Build history of the part. All positions in model axes, mm. A direction names the side the tool comes from. Round coordinates to 2 decimals unless told otherwise and drop trailing zeros. Write each loop counter-clockwise with the first axis right and the second up, starting at its lowest first coordinate (ties: lowest second). Pieces come first, ordered by that corner, then holes. Notation, with made-up numbers: (-35.5, -20.5) - (2.5, -20.5) arc R23 ccw to (2.5, 9.5) - close; hole circle Ø1 at (33, 21.5). An arc over 180 degrees is marked (long way). Write each question's results on one line, items separated by ' | '.
from build123d import *

# Parameters (mm, degrees)
F0_W     = 62
F0_H     = 62
F1_DEPTH = 2
F0_W_2   = 65
F0_H_2   = 65
F2_DEPTH = 50
F3_R     = 2
F4_R     = 1.8
F5_DEPTH = 25
F6_DEPTH = 25
F4_R_2   = 2.55
F7_DEPTH = 5


# Not quite as in the source:
# - a fillet or chamfer that OpenCascade refuses, or shapes differently, is made with other operations: its cross-section is extruded or revolved along the edge and cut away or added


with BuildPart() as f1:
    # F0 (on Front) → F1 (new body)
    with BuildSketch(Plane.XZ):
        with Locations((-0.6578962505, -3.6181825721)):
            Rectangle(F0_W, F0_H)
    extrude(amount=F1_DEPTH)

    # F0 (on Front) → F2 (join)
    with BuildSketch(Plane.XZ):
        with Locations((-0.6578962505, -3.6181825721)):
            Rectangle(F0_W_2, F0_H_2)
        with Locations((-0.6578962505, -3.6181825721)):
            Rectangle(F0_W, F0_H, mode=Mode.SUBTRACT)
    extrude(amount=F2_DEPTH)

    # F3
    f3_edges = [f1.edges().sort_by_distance(p)[0] for p in [
        (31.842104, 0, -3.618183),
        (-0.657896, 0, 28.881817),
        (-33.157896, 0, -3.618183),
        (-0.657896, 0, -36.118183),
        (31.842104, -25, 28.881817),
        (31.842104, -25, -36.118183),
        (-33.157896, -25, -36.118183),
        (-33.157896, -25, 28.881817),
    ]]
    fillet(f3_edges, radius=F3_R)

    # F4 (on face) → F5 (cut)
    with BuildSketch(Plane.YZ.offset(31.8421037495)):
        with Locations((-26, 21.3318174279)):
            Circle(F4_R)
    extrude(amount=-F5_DEPTH, mode=Mode.SUBTRACT)

    # F4 (on face) → F6 (cut)
    with BuildSketch(Plane.YZ.offset(31.8421037495)):
        with Locations((-26, 13.2318174279)):
            Circle(F4_R)
        with Locations((-26, 5.1318174279)):
            Circle(F4_R)
    extrude(amount=-F6_DEPTH, mode=Mode.SUBTRACT)

    # F4 (on face) → F7 (join)
    with BuildSketch(Plane.YZ.offset(31.8421037495)):
        with Locations((-26, 21.3318174279)):
            Circle(F4_R_2)
        with Locations((-26, 21.3318174279)):
            Circle(F4_R, mode=Mode.SUBTRACT)
        with Locations((-26, 13.2318174279)):
            Circle(F4_R_2)
        with Locations((-26, 13.2318174279)):
            Circle(F4_R, mode=Mode.SUBTRACT)
        with Locations((-26, 5.1318174279)):
            Circle(F4_R_2)
        with Locations((-26, 5.1318174279)):
            Circle(F4_R, mode=Mode.SUBTRACT)
    extrude(amount=F7_DEPTH)

    # F8: fillet of radius 1 on 3 edges, made by hand

    # F8_s1 → F8_t2 (revolve, cut)
    with BuildSketch(Plane.XY.offset(21.3318174279)):
        with BuildLine():
            ThreePointArc((35.873857913, -23.45), (36.4862303487, -23.659430585), (36.8421037495, -24.2))
            Line((36.8421037495, -24.2), (36.8421037495, -23.45))
            Line((36.8421037495, -23.45), (35.873857913, -23.45))
        make_face()
    revolve(axis=Axis((36.8421037495, -26, 21.3318174279), (1, 0, 0)), mode=Mode.SUBTRACT)

    # F8_s3 → F8_t4 (revolve, cut)
    with BuildSketch(Plane.XY.offset(13.2318174279)):
        with BuildLine():
            ThreePointArc((35.873857913, -23.45), (36.4862303487, -23.659430585), (36.8421037495, -24.2))
            Line((36.8421037495, -24.2), (36.8421037495, -23.45))
            Line((36.8421037495, -23.45), (35.873857913, -23.45))
        make_face()
    revolve(axis=Axis((36.8421037495, -26, 13.2318174279), (1, 0, 0)), mode=Mode.SUBTRACT)

    # F8_s5 → F8_t6 (revolve, cut)
    with BuildSketch(Plane.XY.offset(5.1318174279)):
        with BuildLine():
            ThreePointArc((35.873857913, -23.45), (36.4862303487, -23.659430585), (36.8421037495, -24.2))
            Line((36.8421037495, -24.2), (36.8421037495, -23.45))
            Line((36.8421037495, -23.45), (35.873857913, -23.45))
        make_face()
    revolve(axis=Axis((36.8421037495, -26, 5.1318174279), (1, 0, 0)), mode=Mode.SUBTRACT)


solid = f1.part
(1) Two-plate mould, pull along X, no slides. Class faces 1 (the flat face through (31.842, -26, -4)), 2 (the flat face through (-31.658, -26, -4)), 3 (the cylindrical face through (-0.231, -0.601, -35.548)): released by +X, released by -X, zero draft, split by the parting line, or undercut.
Worked answers:
face 1: released by +X | face 2: undercut | face 3: zero draft
(2) Slice it at B-B, the plane x = -27. Write the cut outline in (y, z), and give its area (3 significant figures).
Worked answers:
outline: (-50, -36.12) - (-2, -36.12) arc R2 ccw to (0, -34.12) - (0, 26.88) arc R2 ccw to (-2, 28.88) - (-50, 28.88) - (-50, 27.38) - (-2, 27.38) - (-2, -34.62) - (-50, -34.62) - close | area: 272 mm2
(3) Tool access for faces 4 (the cylindrical face through (33.83, -28.548, 21.444)), 5 (the cylindrical face through (31.24, -0.57, -3.19)), 6 (the flat face through (-1, -2, -3)): list every direction of +Z, -Z, +X, -X, +Y, -Y with a clear straight run to the whole face (end or side of a thin tool).
Worked answers:
face 4: +X | face 5: +Z, -Z, +X, +Y | face 6: -Y
(4) Slice it at D-D, the plane y = -26. State how many separate pieces and enclosed holes the cut face has, and give its area (3 significant figures).
Worked answers:
separate pieces: 3 | enclosed holes: 0 | area: 383 mm2
(5) Slice it at C-C, the plane z = 1. Write the cut outline in (x, y).
Worked answers:
outline: (-33.16, -50) - (-31.66, -50) - (-31.66, -2) - (30.34, -2) - (30.34, -50) - (31.84, -50) - (31.84, -2) arc R2 ccw to (29.84, 0) - (-31.16, 0) arc R2 ccw to (-33.16, -2) - close
(6) Slice it at A-A, the plane y = -16. Write the cut outline in (x, z), and give its area (3 significant figures).
Worked answers:
outline: (-33.16, -34.12) arc R2 ccw to (-31.16, -36.12) - (29.84, -36.12) arc R2 ccw to (31.84, -34.12) - (31.84, 26.88) arc R2 ccw to (29.84, 28.88) - (-31.16, 28.88) arc R2 ccw to (-33.16, 26.88) - close; hole (-31.66, -34.62) - (30.34, -34.62) - (30.34, 27.38) - (-31.66, 27.38) - close | area: 378 mm2
(7) Drill centre lines: probe 1 along Z at (x, y) = (34.4, -26); probe 2 along X at (y, z) = (-20, 23); probe 3 along Z at (x, y) = (-25.5, -10.5). Where is each one in solid material? Low to high. Write a range as [from, to].
Worked answers:
probe 1: z = [2.58, 3.33], [6.93, 7.68], [10.68, 11.43], [15.03, 15.78], [18.78, 19.53], [23.13, 23.88] | probe 2: x = [-33.16, -31.66], [30.34, 31.84] | probe 3: z = [-36.12, -34.62], [27.38, 28.88]
(8) Flat gauge pins, fed straight in: pin 1 Ø3 at (x, z) = (-3.5, -7) entering from -Y; pin 2 Ø3 at (y, z) = (-26, 5.13) entering from +X; pin 3 Ø6 at (y, z) = (-26, 5.13) entering from +X; pin 4 Ø12 at (y, z) = (-18.5, -21.5) entering from +X. Where does each tip first touch, or does it go through?
Worked answers:
pin 1: stops at y = -2 | pin 2: stops at x = -31.66 | pin 3: stops at x = 36.84 | pin 4: stops at x = 31.84
